Part model, mm, in its own coordinate system. A direction names the side the tool comes from. Give positions to 0.01 mm unless a question says otherwise; leave off trailing zeros. Write each loop counter-clockwise with the first axis right and the second up, starting at its lowest first coordinate (ties: lowest second). Pieces come first, ordered by that corner, then holes. Notation, with made-up numbers: M 4.25,50 L 45.25,50 A3 ccw 45.25,55 Z; hole C 80,86 d5. An arc over 180 degrees is marked long. Use a Markdown table: item, result.
```python
from build123d import *

# Parameters (mm, degrees)
SKETCH1_W           = 50.8
SKETCH1_H           = 50.8
BOSS_EXTRUDE1_DEPTH = 5.08
SKETCH2_R           = 3.048
SKETCH2_W           = 5.08
SKETCH2_H           = 5.08
CUT_EXTRUDE1_DEPTH  = 5.08


with BuildPart() as part:
    # Sketch1 → Boss-Extrude1 (new body)
    with BuildSketch(Plane(origin=(0, 0, 0), x_dir=(1, 0, 0), z_dir=(0, 1, 0))):
        with Locations((9.389105058, -7.511284047)):
            Rectangle(SKETCH1_W, SKETCH1_H)
    extrude(amount=BOSS_EXTRUDE1_DEPTH)

    # Sketch2 → Cut-Extrude1 (cut)
    with BuildSketch(Plane(origin=(0, 5.08, 0), x_dir=(1, 0, 0), z_dir=(0, 1, 0))):
        with Locations(Location((9.389105058, 5.120135953, 0), (0, 0, 270))):
            Circle(SKETCH2_R)
        with Locations((32.249105058, -22.751284047)):
            Rectangle(SKETCH2_W, SKETCH2_H)
        with Locations((-13.470894942, -12.591284047)):
            Rectangle(SKETCH2_W, SKETCH2_H)
        with Locations((-13.470894942, -22.751284047)):
            Rectangle(SKETCH2_W, SKETCH2_H)
        with Locations((32.249105058, -12.591284047)):
            Rectangle(SKETCH2_W, SKETCH2_H)
        with Locations((32.249105058, -2.431284047)):
            Rectangle(SKETCH2_W, SKETCH2_H)
        with Locations((32.249105058, 7.728715953)):
            Rectangle(SKETCH2_W, SKETCH2_H)
        with Locations((-13.470894942, 7.728715953)):
            Rectangle(SKETCH2_W, SKETCH2_H)
        with Locations((-13.470894942, -2.431284047)):
            Rectangle(SKETCH2_W, SKETCH2_H)
    extrude(amount=-CUT_EXTRUDE1_DEPTH, mode=Mode.SUBTRACT)


solid = part.part
```
1. Cut at A-A, the plane z = -7. Give the cut face in (x, y).
Findings below:
| item | result |
|---|---|
| outline | M -10.93,0 L 6.99,0 L 6.99,5.08 L -10.93,5.08 Z; M 11.79,0 L 29.71,0 L 29.71,5.08 L 11.79,5.08 Z |
2. Two-plate mould, pull along Z, no slides. Class faces 4 (the flat face through (-16.011, 3, -14)), 5 (the flat face through (9, 3, -17.889)), 6 (the flat face through (-14, 3, 20.211)): released by +Z, released by -Z, zero draft, split by the parting line, or undercut.
Findings below:
| item | result |
|---|---|
| face 4 | zero draft |
| face 5 | released by -Z |
| face 6 | undercut |
3. Tool access for faces 1 (the flat face through (-16.011, 3, -3)), 2 (the flat face through (32, 3, -0.109)), 3 (the flat face through (-10.931, 3, -8)): list every direction of +Z, -Z, +X, -X, +Y, -Y with a clear straight run to the whole face (end or side of a thin tool).
Findings below:
| item | result |
|---|---|
| face 1 | +Z, -Z, -X, +Y, -Y |
| face 2 | +X, +Y, -Y |
| face 3 | -X, +Y, -Y |
4. Drill centre lines: L1, parallel to Z at x = -11, y = 1.7; L2, parallel to X at y = 3, z = 15; L3, parallel to X at y = 2.55, z = -6. Where is each one in solid material? Low to high.
Findings below:
| item | result |
|---|---|
| L1 | -17.89 to -10.27, -5.19 to -0.11, 4.97 to 10.05, 15.13 to 20.21, 25.29 to 32.91 |
| L2 | -10.93 to 29.71 |
| L3 | -10.93 to 6.47, 12.31 to 29.71 |
5. Cut at C-C, the plane z = 11.5. Give the cut face in (x, y), then the cut area to 3 significant figures.
Findings below:
| item | result |
|---|---|
| outline | M -10.93,0 L 29.71,0 L 29.71,5.08 L -10.93,5.08 Z |
| area | 206 mm2 |
6. Drop a flat-ended pin along its axis: P1, Ø1.5, axis at y = 3, z = 22, coming from the +X side. Give the stop position or say it passes through.
Findings below:
| item | result |
|---|---|
| P1 | x = 29.71 |
7. Cut at B-B, the plane x = 7. Give the cut face in (y, z), then the cut area to 3 significant figures.
Findings below:
| item | result |
|---|---|
| outline | M 0,-17.89 L 5.08,-17.89 L 5.08,-7.01 L 0,-7.01 Z; M 0,-3.23 L 5.08,-3.23 L 5.08,32.91 L 0,32.91 Z |
| area | 239 mm2 |
